Study the drawing (mm; zero at the part's minimum x, y, z) and answer. Give positions to 0.01 mm unless a question says otherwise; leave off trailing zeros. Order: outer loops, then holes, each group sorted by start corner. A loop starts at its lowest first (then second) coordinate and runs counter-clockwise, first axis right, second up. Notation, with made-up numbers: (-27, 53) -> (18, 53) arc R23 cw to (18, 64) -> close; hole circle Ø1 at (-2, 7.25). An arc over 180 degrees is marked (long way). Answer as CSV lines item,"result". Start each with the question number.
1. Find the intervals of material crossed by L1, parallel to X at y = 51.5, z = 0.5; L2, parallel to Y at x = 31, z = 1.1 (1 decimal); L3, parallel to Y at x = 44.5, z = 1.3 (1 decimal), in increasing order.
2. A cutting plane is placed at A-A (y = 23.5). Give the vertices of the cut face in (x, z).
3. A cutting plane is placed at B-B (x = 30). Give the vertices of the cut face in (y, z), then the cut area to 3 significant figures.
4. A cutting plane is placed at C-C (y = 67.5). Give the vertices of the cut face in (x, z).
5. Flat-ended cylindrical pins translate along their axes: pin 1 (5.5 mm diameter, centred on x = 44, y = 51.5, fed in from -Z); pin 2 (2 mm diameter, centred on x = 30, y = 67.5, fed in from +Z). Find the tip coordinate at first contact, or state that the pin passes through.
6. A cutting plane is placed at D-D (z = 0.25). Give the vertices of the cut face in (x, y), then the cut area to 3 significant figures.
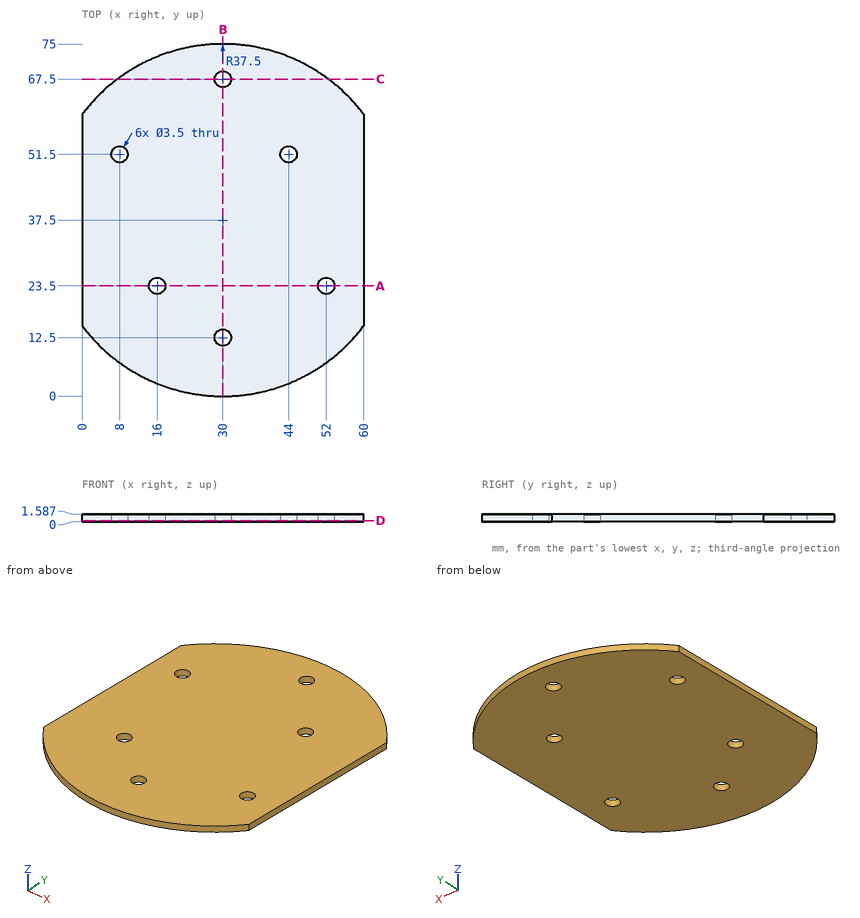
Answer sheet:
1,L1,"x = 0 to 6.25, 9.75 to 42.25, 45.75 to 60"
1,L2,"y = 0 to 11.1, 13.9 to 66.1, 68.9 to 75"
1,L3,"y = 2.9 to 49.8, 53.2 to 72.1"
2,outline,"(0, 0) -> (14.25, 0) -> (14.25, 1.59) -> (0, 1.59) -> close; (17.75, 0) -> (50.25, 0) -> (50.25, 1.59) -> (17.75, 1.59) -> close; (53.75, 0) -> (60, 0) -> (60, 1.59) -> (53.75, 1.59) -> close"
3,outline,"(0, 0) -> (10.75, 0) -> (10.75, 1.59) -> (0, 1.59) -> close; (14.25, 0) -> (65.75, 0) -> (65.75, 1.59) -> (14.25, 1.59) -> close; (69.25, 0) -> (75, 0) -> (75, 1.59) -> (69.25, 1.59) -> close"
3,area,"108 mm^2"
4,outline,"(7.5, 0) -> (28.25, 0) -> (28.25, 1.59) -> (7.5, 1.59) -> close; (31.75, 0) -> (52.5, 0) -> (52.5, 1.59) -> (31.75, 1.59) -> close"
5,pin 1,"stops at z = 0"
5,pin 2,"passes through"
6,outline,"(0, 15) arc R37.5 ccw to (60, 15) -> (60, 60) arc R37.5 ccw to (0, 60) -> close; hole circle Ø3.5 at (8, 51.5); hole circle Ø3.5 at (16, 23.5); hole circle Ø3.5 at (30, 12.5); hole circle Ø3.5 at (30, 67.5); hole circle Ø3.5 at (44, 51.5); hole circle Ø3.5 at (52, 23.5)"
6,area,"3,900 mm^2"
